Autodesk Inventor part; units mm, degrees
ref_plane "Work Plane1" through (3.4, 3.22, 16.2481) normal (0, -0.9654954, 0.2604203) x (-0.7523847, -0.1715451, -0.6359949)
ref_plane "Work Plane4" through (3.4, 1.6696, -10.5) normal (0, -0.9654954, -0.2604203) x (-0.7523847, 0.1715451, -0.6359949)
ref_plane "YZ Plane" through (0, 0, 0) normal (1, 0, 0) x (0, 1, 0)
sketch "Sketch1" plane through (0, 0, 0) normal (0, 1, 0) x (-1, 0, 0)
  circle A0 centre (0, 0) radius 19
  dimension "d0" = 38
extrude "Extrusion1" add sketch "Sketch1" along normal blind 20
sketch "Sketch2" plane through (0, 0, 0) normal (0, -1, 0) x (1, 0, 0)
  line L0 (0, -10.5) -> (3.4, -10.5)
  line L1 (3.4, -10.5) -> (3.4, -19)
  line L2 (3.4, -19) -> (0, -19)
  line L3 (0, -19) -> (-3.4, -19)
  line L4 (-3.4, -19) -> (-3.4, -10.5)
  line L5 (-3.4, -10.5) -> (0, -10.5)
  point P0 (0, 0)
  dimension "d3" = 10.5
  dimension "d5" = 8.5
  dimension "d113" = 3.4
  dimension "d114" = 3.4
sketch "Sketch3" plane through (0, 0, 0) normal (0, -1, 0) x (1, 0, 0)
  line L0 (0.251, 10.5) -> (3.4, 10.5)
  line L1 (3.4, 10.5) -> (3.4, 19)
  line L2 (3.4, 19) -> (-0.351, 19)
  line L3 (-0.351, 19) -> (-3.4, 19)
  line L4 (-3.4, 19) -> (-3.4, 10.5)
  line L5 (-3.4, 10.5) -> (0.251, 10.5)
  point P0 (0, 0)
  dimension "d22" = 8.5
  dimension "d106" = 10.5
  dimension "d107" = 3.4
  dimension "d110" = 3.4
extrude "Extrusion2" cut sketch "Sketch3" against normal blind 3.22
extrude "Extrusion3" cut sketch "Sketch2" against normal blind 3.22
sketch "Sketch4" plane through (0, 0, 0) normal (1, 0, 0) x (0, 1, 0)
  line L0 (0, -10.5) -> (3.22, -10.5)
  line L1 (3.22, -10.5) -> (3.22, -16.6)
  line L2 (3.22, -10.5) -> (3.22, -18.6933)
  line L3 (3.22, -16.6) -> (3.22, -10.5)
  line L4 (3.22, -10.5) -> (1.52, -10.5)
  line L5 (1.52, -10.5) -> (3.22, -16.6)
  line L6 (-0.644, 0) -> (3.864, 0)
  point P0 (0, 0)
  dimension "d28" = 6.1
  dimension "d29" = 1.7
revolve "Revolution1" add sketch "Sketch4" angle 360 about axis through (0, -10, 0) along (0, 1, 0)
sketch "Sketch5" plane through (0, 20, 0) normal (0, 1, 0) x (1, 0, 0)
  circle A0 centre (0, 0) radius 4.81
  dimension "d31" = 9.62
extrude "Extrusion4" cut sketch "Sketch5" against normal through all
sketch "Sketch6" plane through (0, 0, 0) normal (1, 0, 0) x (0, 1, 0)
  line L0 (0, -4.81) -> (13.0829, -17.01)
  line L1 (20, -19) -> (20, 19)
  line L2 (13.0829, -4.81) -> (0, -4.81)
  line L3 (-2.6166, 0) -> (15.6995, 0)
  line L4 (13.0829, -4.81) -> (13.0829, -17.01)
  line L5 (3.22, -19) -> (20, -19)
  line L6 (0, -4.81) -> (13.0829, -4.81) construction
  point P0 (0, 0)
  point P1 (20, -4.81)
  point P2 (13.0829, -17.01)
  dimension "d85" = 12.2
  dimension "d90" = 13.0829
revolve "Revolution2" cut sketch "Sketch6" angle 360 about axis through (0, -10, 0) along (0, 1, 0)
ref_plane "Work Plane1" through (3.4, 3.22, 16.2481) normal (0, -0.9654954, 0.2604203) x (-0.7523847, -0.1715451, -0.6359949)
sketch "Sketch10" plane through (3.4, 3.22, 16.2481) normal (0, -0.9654954, 0.2604203) x (-0.7523847, -0.1715451, -0.6359949)
  line L0 (9.3243, 0.3271) -> (9.0379, 0)
  line L1 (-1.5552, -1.7763) -> (0, 0)
  line L2 (9.0379, 0) -> (0, 0)
  circle A0 centre (4.519, 0) radius 2
  point P0 (13.4442, 10.1942)
  dimension "d111" = 4
extrude "Extrusion5" cut sketch "Sketch10" along normal mid plane 4
ref_plane "Work Plane4" through (3.4, 1.6696, -10.5) normal (0, -0.9654954, -0.2604203) x (-0.7523847, 0.1715451, -0.6359949)
sketch "Sketch12" plane through (3.4, 1.6696, -10.5) normal (0, -0.9654954, -0.2604203) x (-0.7523847, 0.1715451, -0.6359949)
  line L0 (-0.2864, -0.3271) -> (0, 0)
  ellipse E0 centre (-3.8539, -9.5633) end of major axis (8.6357, -20.4981) minor radius 16.0272 (9.0379, 0) -> (3.9217, 4.4793) ccw
  line L1 (0, 0) -> (3.9217, 4.4793)
  line L2 (4.8298, -4.8065) -> (5.1162, -4.4793)
  line L3 (5.1162, -4.4793) -> (3.9217, 4.4793)
  line L4 (10.5931, 1.7763) -> (9.0379, 0)
  line L5 (9.0379, 0) -> (0, 0)
  circle A0 centre (4.519, 0) radius 2
  point P0 (-4.4062, -10.1942)
  point P1 (4.519, 0)
  dimension "d116" = 4
extrude "Extrusion6" cut sketch "Sketch12" along normal mid plane 4 contours A0 L3 L5 | L5 L3 A0 | L3 L5 A0 | L3 A0 L5
sketch "Sketch18" plane through (0, 0, 0) normal (0.1099078, 0, 0.9939418) x (0.9939418, 0, -0.1099078)
  line L0 (19, 20) -> (-19, 20)
  line L1 (19, 0) -> (5.4339, 0)
  line L2 (4.5334, 0) -> (5.4339, 0)
  line L3 (5.4339, 0) -> (19, 12.6506)
  line L4 (19, 0) -> (19, 20)
  line L5 (5.4339, 0) -> (23.9832, 0) construction
  line L6 (1.3249, 0) -> (19, 0)
  line L7 (19, 12.6506) -> (19, 0)
  line L8 (19, 0) -> (19, 20)
  line L9 (19, 0) -> (5.4339, 0)
  point P0 (0, 0)
  point P1 (24.4257, 20)
  dimension "d91" = 43
sketch "Sketch20" plane through (0, 0, 0) normal (-0.1099078, 0, 0.9939418) x (0.9939418, 0, 0.1099078)
  line L0 (5.4339, 3.22) -> (5.4339, 0)
  line L1 (5.4339, 0) -> (19, 12.6506)
  line L2 (19, 0) -> (19, 20)
  line L3 (5.4339, 0) -> (23.9832, 0) construction
  line L4 (1.3249, 0) -> (19, 0)
  line L5 (19, 12.6506) -> (19, 0)
  line L6 (5.4339, 0) -> (4.5334, 0)
  line L7 (19, 0) -> (5.4339, 0)
  point P0 (0, 0)
  point P1 (10.438, 5)
  point P2 (-18.8849, 20)
  point P3 (-18.8849, 20)
  dimension "d94" = 43
sketch "Sketch21" plane through (0, 0, 0) normal (-0.1099078, 0, 0.9939418) x (0.9939418, 0, 0.1099078)
  point P0 (0, 0)
sketch "Sketch22" plane through (0, 0, 0) normal (-0.1099078, 0, 0.9939418) x (0.9939418, 0, 0.1099078)
  line L0 (-18.8849, 20) -> (-19, 20)
  line L1 (-5.4339, 0) -> (21.9126, 0) construction
  line L2 (-5.4339, 0) -> (-4.5334, 0)
  line L3 (-5.4339, 0) -> (-19, 14.5478)
  line L4 (-19, 0) -> (-19, 20)
  line L5 (-5.4339, 0) -> (14.4577, 0) construction
  line L6 (-19, 0) -> (-1.3249, 0)
  line L7 (-19, 14.5478) -> (-19, 0)
  line L8 (-19, 0) -> (-5.4339, 0)
  point P0 (0, 0)
  dimension "d97" = 133
sketch "Sketch23" plane through (0, 0, 0) normal (0.1099078, 0, 0.9939418) x (0.9939418, 0, -0.1099078)
  line L0 (-9.5907, 0) -> (-1.3249, 0)
  line L1 (-5.6359, 0) -> (1.2007, 0) construction
  line L2 (-4.5334, 0) -> (-5.4339, 0)
  line L3 (-5.4339, 0) -> (-19, 14.5478)
  line L4 (-19, 0) -> (-19, 20)
  line L5 (-5.4339, 0) -> (14.4577, 0) construction
  line L6 (-19, 0) -> (-1.3249, 0)
  line L7 (-19, 14.5478) -> (-19, 0)
  line L8 (-19, 0) -> (-5.4339, 0)
  point P0 (0, 0)
  point P1 (-18.8849, 20)
  point P2 (-18.8849, 20)
  dimension "d100" = 133
extrude "Extrusion13" cut sketch "Sketch18" along normal through all both and the other way through all
extrude "Extrusion14" cut sketch "Sketch20" along normal through all both and the other way through all
extrude "Extrusion15" cut sketch "Sketch22" along normal through all both and the other way through all
extrude "Extrusion16" cut sketch "Sketch23" along normal through all both and the other way through all
sketch "Sketch25" plane through (0, 20, 0) normal (0, 1, 0) x (1, 0, 0)
  circle A0 centre (0, 0) radius 17
  dimension "d103" = 34
extrude "Extrusion17" cut sketch "Sketch25" against normal blind 6.92
properties part number "LightShieldBottom" material "Glass"
Source: CAD feature listing. Evaluate the final solid. Frame: model axes, mm. A direction names the side the tool comes from. Give positions to 0.01 mm unless a question says otherwise; leave off trailing zeros. Write each loop counter-clockwise with the first axis right and the second up, starting at its lowest first coordinate (ties: lowest second). Pieces come first, ordered by that corner, then holes. Notation, with made-up numbers: M 29.5,75 L 47.5,75 A24 cw 47.5,112 Z; hole C 16.25,50 d8. An arc over 180 degrees is marked long. Return JSON: item names as keys, results as strings. Group by question number.
1) Pull-direction query (Z, two-part tool) for faces 6 (the face through (-1.751, 2.004, 12.111)), 7 (the face through (0.039, 4.377, 12.85)), 8 (the face through (0, 3.22, 18)); classes: pulls with the +Z half, pulls with the -Z half, needs draft (parallel to the pull), parting line crosses it, or undercut.
2) Material intervals for line 1 along Z through (x, y) = (0, 17.75); line 2 along X through (y, z) = (1, -1); line 3 along Z through (x, y) = (-9, 14), sorted ascending. Write a range as [from, to].
3) Pin query (flat end, axial travel): P1, Ø3.5, axis at y = 1, z = -15, coming from the +X side; P2, Ø3, axis at x = 3.5, y = 18, coming from the -Z side; P3, Ø0.5, axis at x = -1.5, y = 1, coming from the +Z side. Return the tip coordinate at first contact, or that it passes through.
4) Cut plane B-B, the plane y = 8.5. Output: boundary loops of the cut face in (x, z).
5) Set-up query: faces 1 (the face through (0.04, 4.38, -12.86)), 2 (the face through (9.139, 16.59, -14.334)), 3 (the face through (-3.4, 1, -15)), 4 (the face through (14, 20, -10)), 5 (the face through (3.4, 1, 15)). Return all of +Z, -Z, +X, -X, +Y, -Y with unobstructed straight access to the full face (end or side cutting, diameter ignored); none if empty.
Recorded:
{
 "1": {"face 6": "pulls with the +Z half", "face 7": "undercut", "face 8": "needs draft"},
 "2": {"line 1": "z = [-19, -17], [17, 19]", "line 2": "x = [-6.29, -5.65], [5.65, 6.44]", "line 3": "z = [-16.73, -14.42], [14.42, 16.73]"},
 "3": {"P1": "stops at x = 6.79", "P2": "stops at z = -18.89", "P3": "stops at z = 10.5"},
 "4": {"outline": "M -13.44,0 L -11.79,-14.9 A19 ccw 13.12,-13.74 L 14.64,0 L 13.12,13.74 A19 ccw -11.79,14.9 Z; hole C 0,0 d25.47"},
 "5": {"face 1": "none", "face 2": "+Y", "face 3": "-Z, -Y", "face 4": "+Z, -Z, +X, -X, +Y", "face 5": "+Z, -Y"}
}
